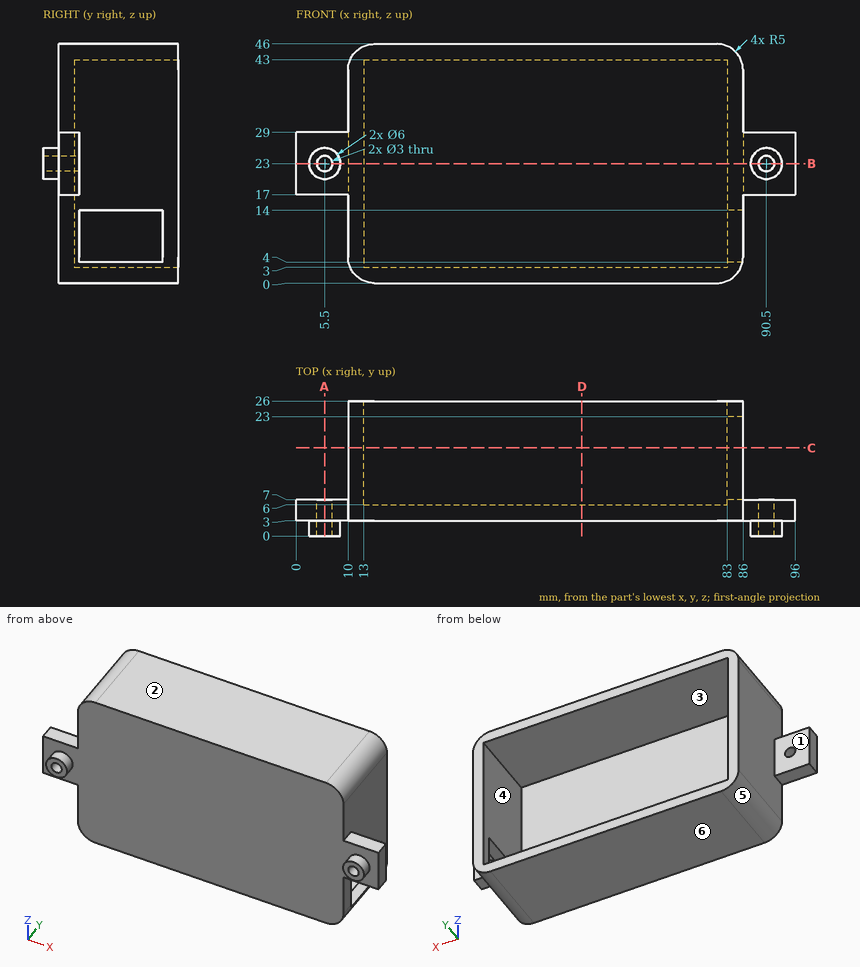
Drawing for the job (mm, zero at the part's lowest x, y, z). A direction names the side the tool comes from. Give positions to 0.01 mm unless a question says otherwise; leave off trailing zeros. Order: outer loops, then holes, each group sorted by start corner. A loop starts at its lowest first (then second) coordinate and runs counter-clockwise, first axis right, second up. Notation, with made-up numbers: M 28,-6 L 87,-6 A23 ccw 87,12 Z; hole C 88,16.25 d2. An arc over 180 degrees is marked long. Use a Markdown table: item, result. Add a question column.
(1) Mould opens along X. For the marked faces 4, 5 and 6 say: +X half, -X half, draft (parallel to the pull), parting line (faces both ways), or undercut.
(2) Saw through at D-D, the plane x = 55. Give the cut face in (y, z), and give its area (3 significant figures).
(3) Saw through at B-B, the plane z = 23. Give the cut face in (x, y).
(4) Drop flat-ended pins along their axis: P1, Ø1, axis at y = 17.5, z = 39.5, coming from the +X side; P2, Ø10, axis at y = 8, z = 24.5, coming from the +X side; P3, Ø6, axis at y = 20.5, z = 25.5, coming from the -X side; P4, Ø6, axis at x = 34, z = 20.5, coming from the +Y side. Give the stop position or say it passes through.
(5) 3-axis set-ups, long thin cutter, end or side, ignore diameter. For the marked faces 1, 2 and 3: which of +Z, -Z, +X, -X, +Y, -Y reach the whole face in a straight line?
(6) Saw through at C-C, the plane y = 17. Give the cut face in (x, z), and give its area (3 significant figures).
(7) Saw through at A-A, the plane x = 5.5. Give the cut face in (y, z).
(8) Probe line 1 along X through (y, z) = (5.5, 23); line 2 along Z through (x, y) = (61, 21.75); line 3 along Z through (x, y) = (5.5, 4.5). List the from-to ranges inside material, lowest first. Write a range as [from, to].
Answer key:
| question | item | result |
|---|---|---|
| 1 | face 4 | undercut |
| 1 | face 5 | -X half |
| 1 | face 6 | draft |
| 2 | outline | M 3,0 L 26,0 L 26,3 L 6,3 L 6,43 L 26,43 L 26,46 L 3,46 Z |
| 2 | area | 258 mm^2 |
| 3 | outline | M 0,3 L 2.5,3 L 2.5,0 L 4,0 L 4,7 L 0,7 Z; M 7,0 L 8.5,0 L 8.5,3 L 87.5,3 L 87.5,0 L 89,0 L 89,7 L 86,7 L 86,26 L 83,26 L 83,6 L 13,6 L 13,26 L 10,26 L 10,7 L 7,7 Z; M 92,0 L 93.5,0 L 93.5,3 L 96,3 L 96,7 L 92,7 Z |
| 4 | P1 | x = 86 |
| 4 | P2 | x = 96 |
| 4 | P3 | x = 10 |
| 4 | P4 | y = 6 |
| 5 | face 1 | +Z, -Z, -X, +Y |
| 5 | face 2 | +Z, +X, -X, +Y, -Y |
| 5 | face 3 | +Y |
| 6 | outline | M 10,5 A5 ccw 15,0 L 81,0 A5 ccw 85.9,4 L 83,4 L 83,3 L 13,3 L 13,43 L 83,43 L 83,14 L 86,14 L 86,41 A5 ccw 81,46 L 15,46 A5 ccw 10,41 Z |
| 6 | area | 645 mm^2 |
| 7 | outline | M 0,20 L 3,20 L 3,17 L 7,17 L 7,21.5 L 0,21.5 Z; M 0,24.5 L 7,24.5 L 7,29 L 3,29 L 3,26 L 0,26 Z |
| 8 | line 1 | [0, 4], [7, 89], [92, 96] |
| 8 | line 2 | [0, 3], [43, 46] |
| 8 | line 3 | [17, 21.5], [24.5, 29] |
